Model file for the job. Use its own axes, mm. Face numbers are marked on the shaded views. A direction names the side the tool comes from. Round coordinates to 2 decimals unless told otherwise and drop trailing zeros. Order: outer loops, then holes, each group sorted by start corner. A loop starts at its lowest first (then second) coordinate and runs counter-clockwise, first axis right, second up. Notation, with made-up numbers: (7.25, 20.5) -> (23.25, 20.5) arc R24 cw to (23.25, 36.5) -> close; hole circle Ø3 at (2.25, -9.5). An arc over 180 degrees is marked (long way). Use CSV: the item, a comma, the result in double quotes.
```python
from build123d import *

# Parameters (mm, degrees)
BOSS_EXTRUDE1_DEPTH = 180.34
SKETCH2_R           = 38.1
CUT_EXTRUDE1_DEPTH  = 101.6
SKETCH3_R           = 61.722
CUT_EXTRUDE2_DEPTH  = 50.8
SKETCH4_R           = 61.722
CUT_EXTRUDE3_DEPTH  = 50.8


with BuildPart() as part:
    # Sketch1 → Boss-Extrude1 (new body)
    with BuildSketch(Plane.XY):
        with BuildLine():
            Line((-95.25, 0), (-95.25, -323.85))
            Line((-95.25, -323.85), (103.886, -323.85))
            Line((103.886, -323.85), (103.886, -247.65))
            Line((103.886, -247.65), (53.086, -247.65))
            Line((53.086, -247.65), (53.086, -79.08501188))
            ThreePointArc((53.086, -79.08501188), (44.811388062, 84.050591907), (-95.25, 0))
        make_face()
    extrude(amount=BOSS_EXTRUDE1_DEPTH)

    # Sketch2 → Cut-Extrude1 (cut)
    with BuildSketch(Plane(origin=(0, 0, 0), x_dir=(-1, 0, 0), z_dir=(0, 0, -1))):
        Circle(SKETCH2_R)
    extrude(amount=-CUT_EXTRUDE1_DEPTH, mode=Mode.SUBTRACT)

    # Sketch3 → Cut-Extrude2 (cut)
    with BuildSketch(Plane.XZ.offset(323.85)):
        with Locations(Location((4.318, 90.17, 0), (0, 0, 270))):
            Circle(SKETCH3_R)
    extrude(amount=-CUT_EXTRUDE2_DEPTH, mode=Mode.SUBTRACT)

    # Sketch4 → Cut-Extrude3 (cut)
    with BuildSketch(Plane.ZY.offset(95.25)):
        with Locations(Location((90.17, -209.55, 0), (0, 0, 270))):
            Circle(SKETCH4_R)
        with Locations(Location((90.17, -9.906, 0), (0, 0, 270))):
            Circle(SKETCH4_R)
    extrude(amount=-CUT_EXTRUDE3_DEPTH, mode=Mode.SUBTRACT)


solid = part.part
```
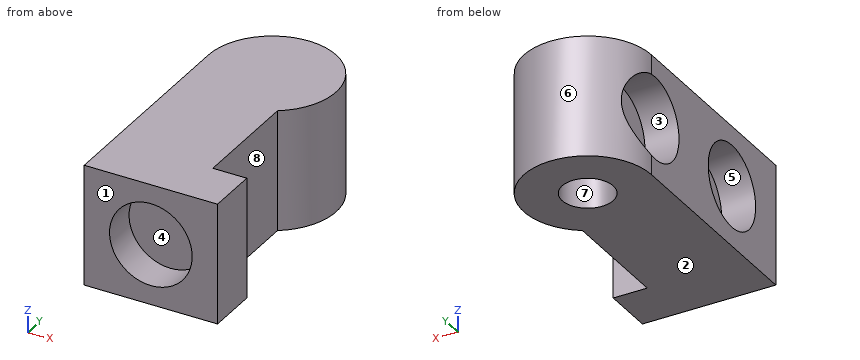
Q1. Mould opens along Z. For the marked faces 1, 2 and 3 say: +Z half, -Z half, draft (parallel to the pull), parting line (faces both ways), or undercut.
From the geometry:
face 1,"draft"
face 2,"-Z half"
face 3,"undercut"
Q2. Cut at A-A (z = 90.17). Give the cut face in (x, y).
From the geometry:
outline,"(-95.25, -323.85) -> (-57.4, -323.85) -> (-57.4, -273.05) -> (66.04, -273.05) -> (66.04, -323.85) -> (103.89, -323.85) -> (103.89, -247.65) -> (53.09, -247.65) -> (53.09, -79.09) arc R95.25 ccw (long way) to (-79.92, 51.82) -> (-44.45, 51.82) -> (-44.45, -71.63) -> (-95.25, -71.63) -> (-95.25, -147.83) -> (-44.45, -147.83) -> (-44.45, -271.27) -> (-95.25, -271.27) -> close; hole circle Ø76.2 at (0, 0)"
Q3. Cut at D-D (z = 160.5). Give the cut face in (x, y), plus the area to 3 significant figures.
From the geometry:
outline,"(-95.25, -323.85) -> (103.89, -323.85) -> (103.89, -247.65) -> (53.09, -247.65) -> (53.09, -79.09) arc R95.25 ccw (long way) to (-95.25, 0) -> close"
area,"68,500 mm²"
Q4. Probe line 1 along X through (y, z) = (-297, 90); line 2 along Y through (x, z) = (0, 25.5); line 3 along Z through (x, y) = (-59, -209.55). List the from-to ranges inside material, lowest first.
From the geometry:
line 1,"x = -95.25 to -57.4, 66.04 to 103.89"
line 2,"y = -323.85 to -38.1, 38.1 to 95.25"
line 3,"z = 0 to 28.45, 151.89 to 180.34"
Q5. Cut at B-B (y = -209.55). Give the cut face in (x, z), plus the area to 3 significant figures.
From the geometry:
outline,"(-95.25, 0) -> (53.09, 0) -> (53.09, 180.34) -> (-95.25, 180.34) -> (-95.25, 151.89) -> (-44.45, 151.89) -> (-44.45, 28.45) -> (-95.25, 28.45) -> close"
area,"20,500 mm²"
Q6. Cut at C-C (x = 59). Give the cut face in (y, z).
From the geometry:
outline,"(-323.85, 0) -> (-247.65, 0) -> (-247.65, 180.34) -> (-323.85, 180.34) -> (-323.85, 118.8) -> (-273.05, 118.8) -> (-273.05, 61.54) -> (-323.85, 61.54) -> close; (-74.78, 0) -> (74.78, 0) -> (74.78, 180.34) -> (-74.78, 180.34) -> close"
Q7. Pin check, flat tips, straight feed: pin 1 (4 mm diameter, centred on x = -39, z = 61, fed in from -Y); pin 2 (15 mm diameter, centred on x = 87, z = 66.5, fed in from +Y); pin 3 (8 mm diameter, centred on y = -224, z = 134, fed in from -X). Stop position of each tip, or through.
From the geometry:
pin 1,"stops at y = -273.05"
pin 2,"stops at y = 52.46"
pin 3,"stops at x = -44.45"
Q8. Which spindle directions (+Z, -Z, +X, -X, +Y, -Y) get a long thin tool onto all of the face, cutting with end or side? Do the marked faces 4, 5, 6, 7 and 8. Say none if no direction does.
From the geometry:
face 4,"-Y"
face 5,"-X"
face 6,"+Z, -Z"
face 7,"-Z"
face 8,"+Z, -Z, +X"
